```python
from build123d import *

# Parameters (mm, degrees)
SKETCH1_W                                        = 32
SKETCH1_H                                        = 52
BOSS_EXTRUDE1_DEPTH                              = 9
CUT_EXTRUDE2_DEPTH                               = 58.078892771
F_10_0_10_DIAMETER_HOLE1_D                       = 10
FILLET3_R                                        = 12
CUT_EXTRUDE3_DEPTH                               = 58.078892771
M4X0_7_TAPPED_HOLE2_D                            = 2.1
M4X0_7_TAPPED_HOLE2_CBORE_D                      = 3.3
M4X0_7_TAPPED_HOLE2_CBORE_DEPTH                  = 2
CBORE_FOR_M3_HEX_HEAD_MACHINE_SCREW5_D           = 3.2
CBORE_FOR_M3_HEX_HEAD_MACHINE_SCREW5_CBORE_D     = 10.2
CBORE_FOR_M3_HEX_HEAD_MACHINE_SCREW5_CBORE_DEPTH = 1
F_4_1_4_1_DIAMETER_HOLE3_D                       = 4.1
CUT_EXTRUDE4_DEPTH                               = 58.078892771
FILLET3_OF_MIRROR11_R                            = 12
CUT_EXTRUDE5_START                               = -9
CUT_EXTRUDE5_OUTLINE_R                           = 5
CUT_EXTRUDE5_OUTLINE_R_2                         = 2.05
CUT_EXTRUDE5_OUTLINE_R_3                         = 1.05
CUT_EXTRUDE5_OUTLINE_R_4                         = 1.6
CUT_EXTRUDE5_DEPTH                               = 9
F_4_1_4_1_DIAMETER_HOLE8_D                       = 4.1
M4X0_7_TAPPED_HOLE3_D                            = 2.1
M4X0_7_TAPPED_HOLE3_CBORE_D                      = 3.3
M4X0_7_TAPPED_HOLE3_CBORE_DEPTH                  = 2


# Read off the part's stored shape, not the designer's step: Cut-Extrude5
with BuildPart() as part:
    # Sketch1 → Boss-Extrude1 (new body)
    with BuildSketch(Plane(origin=(-2, 0, 0), x_dir=(0, -1, 0), z_dir=(-1, 0, 0))):
        with Locations((-8, 25)):
            Rectangle(SKETCH1_W, SKETCH1_H)
    boss_extrude1 = extrude(amount=-BOSS_EXTRUDE1_DEPTH)

    # Sketch3 → Cut-Extrude2 (cut, through all)
    with BuildSketch(Plane(origin=(7, 0, 0), x_dir=(0, 0, -1), z_dir=(1, 0, 0))):
        Polygon((4, 6.75), (-18, 6.75), (-20, 24), (4, 24), align=None)
    cut_extrude2 = extrude(amount=-CUT_EXTRUDE2_DEPTH, mode=Mode.SUBTRACT)

    # Ø10.0 (10) Diameter Hole1 (through all)
    with Locations(Plane.ZY.offset(2)):
        with Locations((28, 0)):
            f_10_0_10_diameter_hole1 = Hole(F_10_0_10_DIAMETER_HOLE1_D / 2)

    # Fillet3
    fillet3_edges = [part.edges().sort_by_distance(p)[0] for p in [
        (2.5, -8, 51),
    ]]
    fillet(fillet3_edges, radius=FILLET3_R)

    # Cut-Sweep1: sweep along a path in Sketch22
    with BuildLine(Plane(origin=(-2, 0, 0), x_dir=(0, -1, 0), z_dir=(-1, 0, 0))) as cut_sweep1_path:
        Line((8, 11), (-6.75, 4.890349955))
    # Sketch21 → Cut-Sweep1 (sweep, cut)
    with BuildSketch(Plane.XZ.offset(8)):
        Polygon((7, 7), (5.5, 7), (4, 10), (7, 10), align=None)
        Polygon((1, 10), (-0.5, 7), (-2, 7), (-2, 10), align=None)
    cut_sweep1 = sweep(path=cut_sweep1_path.line, mode=Mode.SUBTRACT)

    # Sketch23 → Cut-Extrude3 (cut, symmetric)
    with BuildSketch(Plane.ZY.offset(2)):
        Polygon((-1, 6.75), (-1, -8), (7, -8), (0.890349955, 6.75), align=None)
    cut_extrude3 = extrude(amount=CUT_EXTRUDE3_DEPTH, both=True, mode=Mode.SUBTRACT)

    # M4x0.7 Tapped Hole2 (through all)
    with Locations(Plane(origin=(-2, 13.349760492, 32.849760492), x_dir=(0, 0, -1), z_dir=(-1, 0, 0))):
        with Locations((0, 0), (-12.75, -7.361215932), (-12.75, 7.361215932)):
            CounterBoreHole(M4X0_7_TAPPED_HOLE2_D / 2, M4X0_7_TAPPED_HOLE2_CBORE_D / 2, M4X0_7_TAPPED_HOLE2_CBORE_DEPTH)

    # CBORE for M3 Hex Head Machine Screw5 (through all)
    with Locations(Plane(origin=(7, 13.349760492, 41.349760492), x_dir=(0, 0, 1), z_dir=(1, 0, 0))):
        with Locations((0, 0)):
            cbore_for_m3_hex_head_machine_screw5 = CounterBoreHole(CBORE_FOR_M3_HEX_HEAD_MACHINE_SCREW5_D / 2, CBORE_FOR_M3_HEX_HEAD_MACHINE_SCREW5_CBORE_D / 2, CBORE_FOR_M3_HEX_HEAD_MACHINE_SCREW5_CBORE_DEPTH)

    # Ø4.1 (4.1) Diameter Hole3 (through all)
    with Locations(Plane(origin=(-2, 14, 25.510762466), x_dir=(0, 0, -1), z_dir=(-1, 0, 0))):
        with Locations((0, 0)):
            Hole(F_4_1_4_1_DIAMETER_HOLE3_D / 2)

    # Sketch37 → Cut-Extrude4 (cut, symmetric)
    with BuildSketch(Plane.ZY.offset(2)):
        Polygon((32.919624828, 19.334793219), (41, 24), (20, 24), (19.867875139, 22.860423075), (19.45910646, 19.334793219), align=None)
    cut_extrude4 = extrude(amount=CUT_EXTRUDE4_DEPTH, both=True, mode=Mode.SUBTRACT)

    # Mirror11: Boss-Extrude1, Cut-Extrude2, Ø10.0 (10) Diameter Hole1, Cut-Sweep1, Cut-Extrude3, CBORE for M3 Hex Head Machine Screw5, Cut-Extrude4 across plane
    add(boss_extrude1.mirror(Plane.ZY.offset(2)))
    add(cut_extrude2.mirror(Plane.ZY.offset(2)), mode=Mode.SUBTRACT)
    add(f_10_0_10_diameter_hole1.mirror(Plane.ZY.offset(2)), mode=Mode.SUBTRACT)
    add(cut_sweep1.mirror(Plane.ZY.offset(2)), mode=Mode.SUBTRACT)
    add(cut_extrude3.mirror(Plane.ZY.offset(2)), mode=Mode.SUBTRACT)
    add(cbore_for_m3_hex_head_machine_screw5.mirror(Plane.ZY.offset(2)), mode=Mode.SUBTRACT)
    add(cut_extrude4.mirror(Plane.ZY.offset(2)), mode=Mode.SUBTRACT)

    # Fillet3 of Mirror11
    fillet3_of_mirror11_edges = [part.edges().sort_by_distance(p)[0] for p in [
        (-6.5, -8, 51),
    ]]
    fillet(fillet3_of_mirror11_edges, radius=FILLET3_OF_MIRROR11_R)

    # Cut-Extrude5 outline → Cut-Extrude5 (cut)
    with BuildSketch(Plane(origin=(7, 0, 0), x_dir=(0, 0, -1), z_dir=(1, 0, 0)).offset(CUT_EXTRUDE5_START)):
        with BuildLine():
            Line((-32.919624828, 19.334793219), (-41, 24))
            Line((-41, 24), (-51, 24))
            Line((-51, 24), (-51, 4))
            ThreePointArc((-51, 4), (-47.485281374, -4.485281374), (-39, -8))
            Line((-39, -8), (-7, -8))
            Line((-7, -8), (-0.890349955, 6.75))
            Line((-0.890349955, 6.75), (-18, 6.75))
            Line((-18, 6.75), (-19.45910646, 19.334793219))
            Line((-19.45910646, 19.334793219), (-32.919624828, 19.334793219))
        make_face()
        with Locations((-28, 0)):
            Circle(CUT_EXTRUDE5_OUTLINE_R, mode=Mode.SUBTRACT)
        with Locations((-25.510762466, 14)):
            Circle(CUT_EXTRUDE5_OUTLINE_R_2, mode=Mode.SUBTRACT)
        with Locations((-45.599760492, 5.98854456)):
            Circle(CUT_EXTRUDE5_OUTLINE_R_3, mode=Mode.SUBTRACT)
        with Locations((-41.349760492, 13.349760492)):
            Circle(CUT_EXTRUDE5_OUTLINE_R_4, mode=Mode.SUBTRACT)
        with Locations((-32.849760492, 13.349760492)):
            Circle(CUT_EXTRUDE5_OUTLINE_R_3, mode=Mode.SUBTRACT)
        with Locations((-45.599760492, 20.710976424)):
            Circle(CUT_EXTRUDE5_OUTLINE_R_3, mode=Mode.SUBTRACT)
    extrude(amount=CUT_EXTRUDE5_DEPTH, mode=Mode.SUBTRACT)

    # Ø4.1 (4.1) Diameter Hole8 (through all)
    with Locations(Plane(origin=(-2, 14, 25.510762466), x_dir=(0, 0, 1), z_dir=(1, 0, 0))):
        with Locations((0, 0)):
            Hole(F_4_1_4_1_DIAMETER_HOLE8_D / 2)

    # M4x0.7 Tapped Hole3 (through all)
    with Locations(Plane(origin=(-2, 13.349760492, 32.849760492), x_dir=(0, 0, 1), z_dir=(1, 0, 0))):
        with Locations((0, 0), (12.75, -7.361215932), (12.75, 7.361215932)):
            CounterBoreHole(M4X0_7_TAPPED_HOLE3_D / 2, M4X0_7_TAPPED_HOLE3_CBORE_D / 2, M4X0_7_TAPPED_HOLE3_CBORE_DEPTH)


solid = part.part
```
CAD build for the part. Positions are in the model's coordinates, mm. A direction names the side the tool comes from. Give positions to 0.01 mm unless a question says otherwise; leave off trailing zeros. Write each loop counter-clockwise with the first axis right and the second up, starting at its lowest first coordinate (ties: lowest second). Pieces come first, ordered by that corner, then holes. Notation, with made-up numbers: M -34,-31.5 L -29,-31.5 A21 cw -29,1.5 Z; hole C -20.5,-8 d6. An arc over 180 degrees is marked long. Return JSON: item names as keys, results as strings. Group by question number.
(1) Band-saw the part on C-C (z = 42). Give the cut face in (x, y).
(2) Band-saw the part on D-D (x = -7.5). Give the cut face in (y, z).
(3) Mould opens along Z. For faces 4 (the face through (-11, 5, 33)), 5 (the face through (-6.56, -4.58, 47.39)), 6 (the face through (-7.549, 19.826, 45.035)) say: pulls with the +Z half, pulls with the -Z half, needs draft (parallel to the pull), parting line crosses it, or undercut.
(4) 3-axis set-ups, long thin cutter, end or side, ignore diameter. For faces 1 (the face through (-4, 13, 34)), 2 (the face through (-6, 14, 51)), 3 (the face through (-9.52, -0.52, 6.9)): which of +Z, -Z, +X, -X, +Y, -Y reach the whole face in a straight line?
(5) Flat gauge pins, fed straight in: pin 1 Ø3.5 at (y, z) = (14, 25.51) entering from -X; pin 2 Ø3 at (y, z) = (5.99, 45.6) entering from +X; pin 3 Ø2.5 at (y, z) = (5.99, 45.6) entering from -X. Where does each tip first touch, or does it go through?
(6) Band-saw the part on A-A (x = -4.5). Give the cut face in (y, z), and give its area (3 significant figures).
(7) Band-saw the part on B-B (y = -4.5). Give the cut face in (x, z), and give its area (3 significant figures).
(8) Drill centre lines: L1, parallel to Z at x = -4.5, y = 0; L2, parallel to Z at x = -3.75, y = 1.5; L3, parallel to X at y = 16.5, z = 38.5. Where is each one in solid material? Low to high. Write a range as [from, to].
Entries:
{
 "1": {"outline": "M -11,-7.62 L -2,-7.62 L -2,11.89 L -10,11.89 L -10,8.29 L -11,8.29 Z; M -11,18.41 L -10,18.41 L -10,14.81 L -2,14.81 L -2,24 L -11,24 Z"},
 "2": {"outline": "M -8,7 L 6.75,0.89 L 6.75,18 L 19.33,19.46 L 19.33,32.92 L 24,41 L 24,51 L 4,51 A12 ccw -8,39 Z; hole C 0,28 d10; hole C 5.99,45.6 d2.1; hole C 13.35,41.35 d3.2; hole C 14,25.51 d4.1; hole C 13.35,32.85 d2.1; hole C 20.71,45.6 d2.1"},
 "3": {"face 4": "needs draft", "face 5": "pulls with the +Z half", "face 6": "undercut"},
 "4": {"face 1": "+X", "face 2": "+Z, +X, -X, +Y, -Y", "face 3": "-X"},
 "5": {"pin 1": "passes through", "pin 2": "stops at x = -4", "pin 3": "stops at x = -11"},
 "6": {"outline": "M -8,7 L 6.75,0.89 L 6.75,2.89 L -8,9 Z; M -8,10 L 6.75,3.89 L 6.75,18 L 19.33,19.46 L 19.33,32.92 L 24,41 L 24,51 L 4,51 A12 ccw -8,39 Z; hole C 0,28 d10; hole C 5.99,45.6 d2.1; hole C 13.35,41.35 d3.2; hole C 14,25.51 d4.1; hole C 13.35,32.85 d2.1; hole C 20.71,45.6 d2.1", "area": "1,010 mm^2"},
 "7": {"outline": "M -11,8.55 L -8,8.55 L -9.5,5.55 L -3.5,5.55 L -5,8.55 L -2,8.55 L -2,25.82 L -11,25.82 Z; M -11,30.18 L -2,30.18 L -2,47.47 L -11,47.47 Z", "area": "325 mm^2"},
 "8": {"L1": "z = [3.69, 5.69], [6.69, 23], [33, 50.31]", "L2": "z = [3.06, 3.56], [6.06, 23.23], [32.77, 50.74]", "L3": "x = [-10, -2]"}
}
